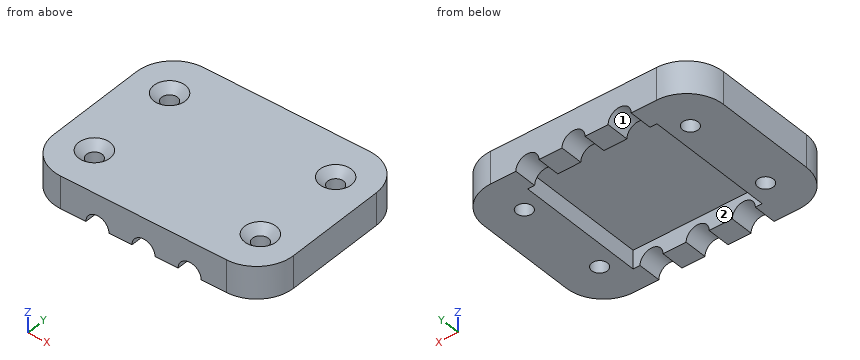
from build123d import *

# Parameters (mm, degrees)
SKETCH_W        = 52
SKETCH_H        = 38
SKETCH_R        = 1.7
PAD_DEPTH       = 7
SKETCH001_R     = 2.5
POCKET_DEPTH    = 38.001
SKETCH002_W     = 28
SKETCH002_H     = 28
POCKET001_DEPTH = 4
FILLET_R        = 8
FILLET001_R     = 8
FILLET002_R     = 8
FILLET003_R     = 8
CHAMFER_SIZE    = 1.7
CHAMFER001_SIZE = 1.7
CHAMFER002_SIZE = 1.7
CHAMFER003_SIZE = 1.7


with BuildPart() as part:
    # Sketch → Pad (new body)
    with BuildSketch(Plane.XY):
        Rectangle(SKETCH_W, SKETCH_H)
        with Locations((-18, 10)):
            Circle(SKETCH_R, mode=Mode.SUBTRACT)
        with Locations((18, 10)):
            Circle(SKETCH_R, mode=Mode.SUBTRACT)
        with Locations((-18, -10)):
            Circle(SKETCH_R, mode=Mode.SUBTRACT)
        with Locations((18, -10)):
            Circle(SKETCH_R, mode=Mode.SUBTRACT)
    extrude(amount=PAD_DEPTH)

    # Sketch001 → Pocket (cut, through all)
    with BuildSketch(Plane.XZ.offset(19)):
        with Locations((-10, 0)):
            Circle(SKETCH001_R)
        Circle(SKETCH001_R)
        with Locations((10, 0)):
            Circle(SKETCH001_R)
    extrude(amount=-POCKET_DEPTH, mode=Mode.SUBTRACT)

    # Sketch002 → Pocket001 (cut)
    with BuildSketch(Plane(origin=(0, 0, 0), x_dir=(1, 0, 0), z_dir=(0, 0, -1))):
        Rectangle(SKETCH002_W, SKETCH002_H)
    extrude(amount=-POCKET001_DEPTH, mode=Mode.SUBTRACT)

    # Fillet
    fillet_edges = [part.edges().sort_by_distance(p)[0] for p in [
        (-26, -19, 3.5),
    ]]
    fillet(fillet_edges, radius=FILLET_R)

    # Fillet001
    fillet001_edges = [part.edges().sort_by_distance(p)[0] for p in [
        (-26, 19, 3.5),
    ]]
    fillet(fillet001_edges, radius=FILLET001_R)

    # Fillet002
    fillet002_edges = [part.edges().sort_by_distance(p)[0] for p in [
        (26, 19, 3.5),
    ]]
    fillet(fillet002_edges, radius=FILLET002_R)

    # Fillet003
    fillet003_edges = [part.edges().sort_by_distance(p)[0] for p in [
        (26, -19, 3.5),
    ]]
    fillet(fillet003_edges, radius=FILLET003_R)

    # Chamfer
    chamfer_edges = [part.edges().sort_by_distance(p)[0] for p in [
        (16.3, -10, 7),
    ]]
    chamfer(chamfer_edges, length=CHAMFER_SIZE)

    # Chamfer001
    chamfer001_edges = [part.edges().sort_by_distance(p)[0] for p in [
        (16.3, 10, 7),
    ]]
    chamfer(chamfer001_edges, length=CHAMFER001_SIZE)

    # Chamfer002
    chamfer002_edges = [part.edges().sort_by_distance(p)[0] for p in [
        (-19.7, 10, 7),
    ]]
    chamfer(chamfer002_edges, length=CHAMFER002_SIZE)

    # Chamfer003
    chamfer003_edges = [part.edges().sort_by_distance(p)[0] for p in [
        (-19.7, -10, 7),
    ]]
    chamfer(chamfer003_edges, length=CHAMFER003_SIZE)


solid = part.part
Design review of the part built by this model. Coordinates are the model's own, in mm. Face numbers are marked on the shaded views. A direction names the side the tool comes from. Round coordinates to 2 decimals unless told otherwise and drop trailing zeros. Loops run counter-clockwise (first coordinate to the right, second up) from the corner with the lowest first, then second, coordinate; pieces in that order, holes last. Notation, with made-up numbers: (-14, 9) - (-9, 9) arc R11 ccw to (-9, 23) - close; hole circle Ø1 at (-40, 64.5). An arc over 180 degrees is marked (long way). One line per question, with ' | ' between items.
1. Clearance check with flat-ended pins moving along their axes: P1, Ø5.5, axis at x = -18, y = 10, coming from the +Z side; P2, Ø8.5, axis at x = 1, y = -1.5, coming from the -Z side. State where each tip first meets the part, or that it passes through.
Results are:
P1: stops at z = 6.35 | P2: stops at z = 4
2. We need section A-A, the plane y = 10. State the section outline as (x, z) points.
Results are:
outline: (-26, 0) - (-19.7, 0) - (-19.7, 5.3) - (-21.4, 7) - (-26, 7) - close; (-16.3, 0) - (-14, 0) - (-14, 4) - (14, 4) - (14, 0) - (16.3, 0) - (16.3, 5.3) - (14.6, 7) - (-14.6, 7) - (-16.3, 5.3) - close; (19.7, 0) - (26, 0) - (26, 7) - (21.4, 7) - (19.7, 5.3) - close
3. We need section B-B, the plane x = 0. State the section outline as (y, z) points, and give its area (3 significant figures).
Results are:
outline: (-19, 2.5) - (-14, 2.5) - (-14, 4) - (14, 4) - (14, 2.5) - (19, 2.5) - (19, 7) - (-19, 7) - close | area: 129 mm²
4. For the marked faces 1 and 2, list the 3-axis set-ups (+Z, -Z, +X, -X, +Y, -Y) from which the entire face can be reached by the end or side of a thin tool; tool diameter is ignored.
Results are:
face 1: -Z, +Y, -Y | face 2: -Z
5. We need section D-D, the plane z = 1.75. State how many separate pieces and enclosed holes the cut face has, and give its area (3 significant figures).
Results are:
separate pieces: 6 | enclosed holes: 4 | area: 994 mm²
6. We need section C-C, the plane y = 2.5. State the section outline as (x, z) points, and give its area (3 significant figures).
Results are:
outline: (-26, 0) - (-14, 0) - (-14, 4) - (14, 4) - (14, 0) - (26, 0) - (26, 7) - (-26, 7) - close | area: 252 mm²
7. For L1, parallel to Y at x = -18, z = 1.3; L2, parallel to X at y = 1, z = 2; L3, parallel to X at y = -8.5, z = 6, list the stretches that pass through material, from the lowest coordinate up. Write a range as [from, to].
Results are:
L1: y = [-19, -11.7], [-8.3, 8.3], [11.7, 19] | L2: x = [-26, -14], [14, 26] | L3: x = [-26, -19.87], [-16.13, 16.13], [19.87, 26]
